Autodesk Inventor part; units mm, degrees
ref_plane "Start Plane" through (0, 0, 0) normal (0, 0, 1) x (1, 0, 0)
ref_plane "End Plane" through (0, 0, 113.3811) normal (0, 0, 1) x (1, 0, 0)
ref_plane "Work Plane4" through (-0.0781, -10.0538, 113.3733) normal (0.0025, 0.3181, 0.9481) x (1, -0.0004, -0.0025)
ref_plane "Start Plane" through (0, 0, 0) normal (0, 0, 1) x (1, 0, 0)
ref_plane "End Plane" through (0, 0, 113.3811) normal (0, 0, 1) x (1, 0, 0)
sketch "Sketch" plane through (0, 0, 0) normal (0, 0, 1) x (1, 0, 0)
  line L0 (-10, -7) -> (-10, 7)
  line L1 (-7, 10) -> (7, 10)
  line L2 (10, 7) -> (10, -7)
  line L3 (7, -10) -> (-7, -10)
  arc A0 (-10, -7) -> (-7, -10) centre (-7, -7) ccw
  arc A1 (-7, 10) -> (-10, 7) centre (-7, 7) ccw
  arc A2 (10, 7) -> (7, 10) centre (7, 7) ccw
  arc A3 (7, -10) -> (10, -7) centre (7, -7) ccw
  arc A4 (-7, 8) -> (-8, 7) centre (-7, 7) ccw
  line L4 (-7, 8) -> (7, 8)
  arc A5 (8, 7) -> (7, 8) centre (7, 7) ccw
  line L5 (8, 7) -> (8, -7)
  arc A6 (7, -8) -> (8, -7) centre (7, -7) ccw
  line L6 (7, -8) -> (-7, -8)
  arc A7 (-8, -7) -> (-7, -8) centre (-7, -7) ccw
  line L7 (-8, -7) -> (-8, 7)
  line L8 (0, 14.8698) -> (0, -14.8698) construction
  line L9 (-14.8698, 0) -> (14.8698, 0) construction
  dimension "d7" = 3
  dimension "d10" = 20
  dimension "d11" = 20
  dimension "d12" = 2
  dimension "d15" = 10
  dimension "d16" = 10
extrude "Body" add sketch "Sketch" along normal up to surface (113.3811 mm away) from surface at 0
sketch "Sketch3" plane through (0, 0, 0) normal (0, 0, 1) x (1, 0, 0)
  line L0 (0, 0) -> (10, 0)
ref_plane "Work Plane3" through (0, 0, 0) normal (0, -1, 0) x (1, 0, 0)
sketch "Sketch4" plane through (0, 0, 0) normal (0, -1, 0) x (1, 0, 0)
  line L0 (-2, 0) -> (12, 0)
  line L1 (-2, 113.3811) -> (12, 113.3811)
  dimension "d18" = 113.3811
ref_plane "Work Plane4" through (-0.0781, -10.0538, 113.3733) normal (0.0025, 0.3181, 0.9481) x (1, -0.0004, -0.0025)
split "Split1" plane through (-0.0781, -10.0538, 113.3733) removes the side toward (0.0025, 0.3181, 0.9481)
sketch "Sketch5" plane through (-7, 10, 0) normal (0, 1, 0) x (1, 0, 0)
  circle A0 centre (7.1219, -23.7725) radius 5
  circle A1 centre (7.1219, -23.7725) radius 9 construction
  circle A2 centre (7.1219, -23.7725) radius 7 construction
  line L0 (3.0805, -30.7725) -> (-0.961, -23.7725)
  line L1 (-0.961, -23.7725) -> (3.0805, -16.7725)
  line L2 (3.0805, -16.7725) -> (11.1634, -16.7725)
  line L3 (11.1634, -16.7725) -> (15.2048, -23.7725)
  line L4 (15.2048, -23.7725) -> (11.1634, -30.7725)
  line L5 (11.1634, -30.7725) -> (3.0805, -30.7725)
  line L6 (-3, -112.3746) -> (-3, -107.6775)
  line L7 (-3, 0) -> (-3, -107.6775)
  line L8 (-3, 0) -> (-3, -112.3746)
  line L9 (17, -107.6254) -> (17, -112.3225)
  line L10 (17, 0) -> (17, -112.3225)
  line L11 (17, 0) -> (17, -107.6254)
  line L12 (0, -106.6632) -> (14, -106.6267)
  line L13 (17, 0) -> (17, -112.3225)
  line L14 (17, -8.3733) -> (-3, -8.3733)
  line L15 (-3, 0) -> (17, 0)
  line L16 (17, -32.0389) -> (-3, -32.0389)
  line L17 (12.1219, -23.7725) -> (12.1219, 0)
  line L18 (0, 0) -> (14, 0)
  line L19 (2.1219, 0) -> (2.1219, -24.4296)
  circle A3 centre (7.1219, -55.9225) radius 2.25
  circle A4 centre (7.1219, -55.9225) radius 4.5
  point P0 (7, 0)
  point P1 (7.1219, -30.7725)
  point P2 (0, -33.0389)
  point P3 (-3, -32.0389)
  point P4 (0, -113.3733)
  point P5 (12.7606, -19.5389)
  point P6 (9.7821, -19.5389)
  point P7 (4.4618, -19.5389)
  point P8 (1.4833, -19.5389)
  point P9 (-3, -8.3733)
  point P10 (2.1219, -8.3733)
  point P11 (2.1219, -18.4328)
  point P12 (12.1219, -18.4328)
  point P13 (12.1219, -8.3733)
  point P14 (12.1219, -19.5389)
  point P15 (2.1219, -19.5389)
  dimension "d21" = 14
  dimension "d19" = 18
  dimension "d22" = 1
  dimension "d27" = 9
  dimension "d31" = 105
extrude "Extrusion2" cut sketch "Sketch5" against normal up to surface (18 mm away) contours A0 | L17 L3 L4 L5 L0 L1 L19 A0 | A0 L19 L1 L2 L3 L17 | L17 L14 L10 L16 L7 L19 L1 L0 L5 L4 L3 | L3 L2 L1 L19 L14 L17 | L17 L15 L10 L14 | L14 L19 L15 L17 | L14 L7 L15 L19
sketch "Sketch8" plane through (-7, 10, 106.6632) normal (0, 1, 0) x (1, 0, -0.0026)
  circle A0 centre (7.2542, 50.7219) radius 2.25
  circle A1 centre (7.2542, 50.7219) radius 5
  point P0 (7.278, 106.6446)
  dimension "d28" = 10
extrude "Extrusion4" cut sketch "Sketch8" against normal through all contours A0 | A1
sketch "Sketch9" plane through (-7, 10, 106.6632) normal (0, 1, 0) x (1, 0, 0)
  circle A0 centre (7.1219, 82.8906) radius 5
  line L0 (2.1219, 106.6632) -> (2.1219, 82.2336)
  line L1 (12.1219, 82.8906) -> (12.1219, 106.6632)
  line L2 (17, 98.2899) -> (-3, 98.2899)
  line L3 (-3, 106.6632) -> (-3, -1.0143)
  line L4 (17, 106.6632) -> (17, -0.9622)
  line L5 (17, 74.6243) -> (-3, 74.6243)
  line L6 (17, 106.6632) -> (17, 74.6243)
  line L7 (-3, 74.6243) -> (-3, 106.6632)
  line L8 (17, 98.2899) -> (-3, 98.2899)
  line L9 (17, 106.6632) -> (-3, 106.6632)
  point P0 (2.1219, 82.8906)
  point P1 (2.1219, 98.2899)
  point P2 (12.1219, 98.2899)
extrude "Extrusion5" cut sketch "Sketch9" against normal through all contours A0 | A0 L0 L2 L1 | L2 L0 L9 L1 | L1 L9 L4 L2 | L2 L3 L9 L0
equation "\"d7\" = G_IR"
equation "\"d10\" = G_H"
equation "\"d11\" = G_W"
equation "\"d12\" = G_T"
equation "\"d15\" = 0.5 * d10"
equation "\"d16\" = 0.5 * d11"
equation "\"d3\" = G_L"
equation "\"G_W\" = 20"
equation "\"G_H\" = 20"
equation "\"G_T\" = 2"
equation "\"G_IR\" = 3"
equation "\"G_L\" = d18"
equation "\"G_OFFSET_START\" = 0"
equation "\"G_OFFSET_END\" = 3.38113"
equation "\"d14\" = G_OFFSET_END + B_L"
properties part number "ISO 12633-2 - 20x20x2 - 113,38" material "Steel, Mild"
Geometry check sheet. Reference: the model listing, model coordinates, mm. A direction names the side the tool comes from. Give positions to 0.01 mm unless a question says otherwise; leave off trailing zeros. Loops run counter-clockwise (first coordinate to the right, second up) from the corner with the lowest first, then second, coordinate; pieces in that order, holes last. Notation, with made-up numbers: M -30,30 L 17,30 A27 ccw 17,48 Z; hole C 64.5,-34 d7. An arc over 180 degrees is marked long. Write item = value, one per line.
(1) Sectioned sample at A-A, the plane z = 55. Record the cut outline in (x, y).
Answer below:
outline = M -10,-7 A3 ccw -7,-10 L -4.79,-10 L -4.79,-8 L -7,-8 A1 cw -8,-7 L -8,7 A1 cw -7,8 L -4.79,8 L -4.79,10 L -7,10 A3 ccw -10,7 Z; M 5.04,-10 L 7,-10 A3 ccw 10,-7 L 10,7 A3 ccw 7,10 L 5.04,10 L 5.04,8 L 7,8 A1 cw 8,7 L 8,-7 A1 cw 7,-8 L 5.04,-8 Z
(2) Tool access check on faces 4 (the face through (-9.1, -9.14, 60.14)), 5 (the face through (4.89, 9.01, 54.41)), 6 (the face through (5.122, -9, 16)), 7 (the face through (-8, 0, 72)), 8 (the face through (0, 8.4, 32.039)). Record the directions out of +Z, -Z, +X, -X, +Y, -Y that give a thin tool (end or side, any length) a straight path to the whole face; none if there is none.
Answer below:
face_4 = +Z, -Z, -X, -Y
face_5 = +Y, -Y
face_6 = -Z, +Y, -Y
face_7 = +Z, -Z
face_8 = -Z, +X, -X, +Y
(3) Sectioned sample at D-D, the plane z = 73.5. Record the cut outline in (x, y).
Answer below:
outline = M -10,-7 A3 ccw -7,-10 L 7,-10 A3 ccw 10,-7 L 10,7 A3 ccw 7,10 L -7,10 A3 ccw -10,7 Z; hole M -8,-7 A1 ccw -7,-8 L 7,-8 A1 ccw 8,-7 L 8,7 A1 ccw 7,8 L -7,8 A1 ccw -8,7 Z
(4) Sectioned sample at B-B, the plane x = -5.75. Record the cut outline in (y, z), plus the area to 3 significant figures.
Answer below:
outline = M -10,8.37 L -8,8.37 L -8,112.7 L -10,113.37 Z; M 8,32.04 L 10,32.04 L 10,106.66 L 8,107.33 Z
area = 359 mm2
(5) Release check for a two-part mould opening along Y. For faces 1 (the face through (4.89, -8.99, 54.41)), 2 (the face through (0, -10, 72)), 3 (the face through (0, 8, 69)) record: released by +Y, released by -Y, zero draft, split by the parting line, or undercut.
Answer below:
face_1 = zero draft
face_2 = released by -Y
face_3 = undercut
(6) Sectioned sample at C-C, the plane y = 5.75. Record the cut outline in (x, z).
Answer below:
outline = M -10,32.04 L -8,32.04 L -8,108.09 L -10,108.1 Z; M 8,32.04 L 10,32.04 L 10,108.04 L 8,108.05 Z
(7) Material ranges on line 1 (Y direction, x = 2.75, z = 48.5); line 2 (X direction, y = -7.75, z = 107), recorded low to high. Write a range as [from, to].
Answer below:
line_1 = [-10, -8], [8, 10]
line_2 = [-9.9, -7.66], [7.66, 9.9]
(8) Gauge pin test, flat ends, axial feed: pin 1 Ø8 at (x, y) = (6, -2.5) entering from +Z; pin 2 Ø6 at (x, z) = (0.12, 55.92) entering from -Y; pin 3 Ø1.6 at (y, z) = (-8.5, 17) entering from -X; pin 4 Ø1.6 at (y, z) = (-9, 19) entering from +X. Record the tip position at first contact, or that the pin passes through.
Answer below:
pin_1 = 111.98
pin_2 = through
pin_3 = -9.83
pin_4 = 9.75
